```python
from build123d import *

# Parameters (mm, degrees)
SKETCH1_W           = 25.012643909
SKETCH1_H           = 8.941938647
BOSS_EXTRUDE1_DEPTH = 2


with BuildPart() as part:
    # Sketch1 → Boss-Extrude1 (new body)
    with BuildSketch(Plane(origin=(0, 0, 0), x_dir=(1, 0, 0), z_dir=(0, 1, 0))):
        Polygon((12.244705421, 9.289945609), (66.543678684, 9.289945609), (66.543678684, -18.710054391), (-43.456321316, -18.710054391), (-43.456321316, -1.162360163), (12.148339373, -1.162360163), align=None)
        with Locations((10.851931882, -8.063685007)):
            Rectangle(SKETCH1_W, SKETCH1_H, mode=Mode.SUBTRACT)
    extrude(amount=BOSS_EXTRUDE1_DEPTH)


solid = part.part
```
The listing builds one solid part. Answer for the finished solid, in the listing's coordinates (mm). A direction names the side the tool comes from. Coordinates: 2 decimals unless noted, no trailing zeros. Loops run counter-clockwise (first coordinate to the right, second up) from the corner with the lowest first, then second, coordinate; pieces in that order, holes last. Notation, with made-up numbers: M 7.5,15.5 L 59.5,15.5 A13 cw 59.5,32.5 Z; hole C 76,-25.5 d11. An arc over 180 degrees is marked long. Answer as a JSON object with one key per item and string values. Group by question number.
Item 1: Section D-D (z = -5) is taken. Write down the section's boundary in (x, y), and give its area (3 significant figures).
Item 2: Section C-C (x = 7) is taken. Write down the section's boundary in (y, z), and give its area (3 significant figures).
Item 3: Section B-B (y = 1.4) is taken. Write down the section's boundary in (x, z), and give its area (3 significant figures).
Item 4: Section A-A (z = 9.5) is taken. Write down the section's boundary in (x, y).
Item 5: Each of these flat-tipped pins is pushed along its axis until it touches: P1, Ø1, axis at x = 7.5, y = 1.5, coming from the -Z side; P2, Ø6, axis at x = -25, z = -4, coming from the +Y side. Where does it stop, or does it pass through?
Item 6: Consider L1, parallel to X at y = 1.1, z = 6.5; L2, parallel to Z at x = 6, y = 1.75; L3, parallel to Z at x = 12.5, y = 1.95. Determine where each line is inside the solid, lowest interval first.
Item 7: Which of the six approach directions +Z, -Z, +X, -X, +Y, -Y give full straight-line access (tool end or side, diameter ignored) to faces 4 (the face through (-16, 1, 1.162)), 5 (the face through (11, 1, 12.535)), 6 (the face through (12, 1, 18.71))?
Item 8: Determine the mould class of faces 1 (the face through (66.544, 1, 5)), 2 (the face through (23.358, 1, 8)), 3 (the face through (-43.456, 1, 10)) for opening direction X: +X half, -X half, draft (parallel to the pull), parting line (faces both ways), or undercut.
Solved:
{
 "1": {"outline": "M 12.21,0 L 66.54,0 L 66.54,2 L 12.21,2 Z", "area": "109 mm2"},
 "2": {"outline": "M 0,1.16 L 2,1.16 L 2,3.59 L 0,3.59 Z; M 0,12.53 L 2,12.53 L 2,18.71 L 0,18.71 Z", "area": "17.2 mm2"},
 "3": {"outline": "M -43.46,1.16 L 12.15,1.16 L 12.24,-9.29 L 66.54,-9.29 L 66.54,18.71 L -43.46,18.71 Z; hole M -1.65,3.59 L 23.36,3.59 L 23.36,12.53 L -1.65,12.53 Z", "area": "2,270 mm2"},
 "4": {"outline": "M -43.46,0 L -1.65,0 L -1.65,2 L -43.46,2 Z; M 23.36,0 L 66.54,0 L 66.54,2 L 23.36,2 Z"},
 "5": {"P1": "stops at z = 1.16", "P2": "passes through"},
 "6": {"L1": "x = -43.46 to -1.65, 23.36 to 66.54", "L2": "z = 1.16 to 3.59, 12.53 to 18.71", "L3": "z = -9.29 to 3.59, 12.53 to 18.71"},
 "7": {"face 4": "-Z, -X, +Y, -Y", "face 5": "+Y, -Y", "face 6": "+Z, +X, -X, +Y, -Y"},
 "8": {"face 1": "+X half", "face 2": "undercut", "face 3": "-X half"}
}
